Could you check a few things on this model? Use its own coordinates, in mm. A direction names the side the tool comes from. Coordinates: 2 decimals unless noted, no trailing zeros. Order: outer loops, then holes, each group sorted by start corner. A loop starts at its lowest first (then second) coordinate and runs counter-clockwise, first axis right, second up. Notation, with made-up numbers: (-24, -27) - (20, -27) arc R26 cw to (20, 12) - close; hole circle Ø5 at (72, -33). An arc over 180 degrees is marked (long way). Answer as a JSON object with one key per item and string values. Group by question number.
(1) Will these pins go through, and if not, where does the flat tip stop? P1, Ø1.5, axis at x = -5.5, z = 2, coming from the +Y side; P2, Ø1, axis at x = -5.5, z = -1.5, coming from the +Y side (3 decimals); P3, Ø2, axis at y = -4, z = 1.5, coming from the +X side.
(2) Which directions (+Z, -Z, +X, -X, +Y, -Y) give clear straight access to the entire face, cutting with the end or side of a thin tool? Please do faces 4 (the flat face through (3, -1, -2.5)), 5 (the flat face through (3, 3, -2.4)).
(3) Please list where these lines run through material, in increasing order: probe 1 along Y at (x, z) = (0, -0.5); probe 2 along Z at (x, y) = (-2, -5); probe 3 along Y at (x, z) = (-0.5, 1.4).
(4) We'd pull the mould along X, two halves only. Please class faces 1 (the cylindrical face through (-0.54, -2.44, -0.03)), 2 (the cylindrical face through (-1.73, -7.81, 0.03)), 3 (the flat face through (-4, -6, -2.5)): pulls with the +X half, pulls with the -X half, needs draft (parallel to the pull), parting line crosses it, or undercut.
(5) Imagine slicing it at A-A, the plane z = -0.3. Write out the boundary of the cut face in (x, y).
from build123d import *

# Parameters (mm, degrees)
SKIZZE1_R                       = 8
SKIZZE1_R_2                     = 2.5
AUFSATZ_LINEAR_AUSTRAGEN1_DEPTH = 2.5
SKETCH1_W                       = 2.6
SKETCH1_H                       = 0.1
CHAMFER1_SIZE                   = 0.1


with BuildPart() as part:
    # Skizze1 → Aufsatz-Linear austragen1 (new, symmetric)
    with BuildSketch(Plane.XY):
        Circle(SKIZZE1_R)
        Circle(SKIZZE1_R_2, mode=Mode.SUBTRACT)
    extrude(amount=AUFSATZ_LINEAR_AUSTRAGEN1_DEPTH, both=True)

    # Sketch1 → Cut-Revolve1 (revolve, cut)
    with BuildSketch(Plane(origin=(0, 0, 0), x_dir=(1, 0, 0), z_dir=(0, 1, 0)), mode=Mode.PRIVATE) as cut_revolve1_sk:
        with Locations((5.3, 2.45)):
            Rectangle(SKETCH1_W, SKETCH1_H)
        with Locations((5.3, -2.45)):
            Rectangle(SKETCH1_W, SKETCH1_H)
    revolve(cut_revolve1_sk.sketch.rotate(Axis((0, 0, -2.5), (0, 0, 1)), 180), axis=Axis((0, 0, -2.5), (0, 0, 1)), mode=Mode.SUBTRACT)

    # Chamfer1
    chamfer1_edges = [part.edges().sort_by_distance(p)[0] for p in [
        (6.6, 0, -2.5),
        (4, 0, -2.5),
        (4, 0, 2.5),
        (6.6, 0, 2.5),
        (-8, 0, -2.5),
        (-8, 0, 2.5),
        (-2.5, 0, -2.5),
        (-2.5, 0, 2.5),
    ]]
    chamfer(chamfer1_edges, length=CHAMFER1_SIZE - 0.0001)  # a hair under: the kernel refuses the full size


solid = part.part
Result set:
{
 "1": {"P1": "stops at y = 6.44", "P2": "stops at y = 6.245", "P3": "stops at x = 7.42"},
 "2": {"face 4": "-Z, +X, -X, +Y, -Y", "face 5": "-Z"},
 "3": {"probe 1": "y = -8 to -2.5, 2.5 to 8", "probe 2": "z = -2.4 to 2.4", "probe 3": "y = -7.98 to -2.45, 2.45 to 7.98"},
 "4": {"face 1": "undercut", "face 2": "parting line crosses it", "face 3": "needs draft"},
 "5": {"outline": "circle Ø16 at (0, 0); hole circle Ø5 at (0, 0)"}
}
